```python
from build123d import *

# Parameters (mm, degrees)
SKETCH2_R           = 76.2
BOSS_EXTRUDE2_DEPTH = 76.2


with BuildPart() as part:
    # Sketch2 → Boss-Extrude2 (new body)
    with BuildSketch(Plane.XY):
        Polygon((0, 0), (803.656, 0), (549.615688221, -508), (131.991038362, -508), align=None)
        with Locations(Location((350.334210966, -312.584818641, 0), (0, 0, 180))):
            Circle(SKETCH2_R, mode=Mode.SUBTRACT)
    extrude(amount=BOSS_EXTRUDE2_DEPTH)


solid = part.part
```
Here's how the part is built. I have some questions about the finished solid (model axes, mm). Give positions to 0.01 mm unless a question says otherwise; leave off trailing zeros. Order: outer loops, then holes, each group sorted by start corner. A loop starts at its lowest first (then second) coordinate and runs counter-clockwise, first axis right, second up. Notation, with made-up numbers: (30, 30) - (71, 30) arc R27 ccw to (71, 50) - close; hole circle Ø4 at (73.5, 84.5). An arc over 180 degrees is marked (long way). Answer as a JSON object with one key per item and string values. Group by question number.
Item 1: For P1, Ø10, axis at y = -87, z = 10, coming from the -X side; P2, Ø4, axis at y = -345.5, z = 59, coming from the -X side; P3, Ø12, axis at y = -379, z = 34, coming from the -X side, each with a flat end and sliding along its axis, tell me the tip position at first contact or that it passes through.
Item 2: If we mould it in two halves opening along Y, with no side actions, what happens to faces 1 (the cylindrical face through (410.804, -266.218, 37.567)), 2 (the flat face through (396, 0, 38)), 3 (the flat face through (66.92, -257.56, 37.57))? For each: pulls with the +Y half, pulls with the -Y half, needs draft (parallel to the pull), parting line crosses it, or undercut.
Item 3: If we section it at C-C on x = 685: Please give me the cut outline in (y, z).
Item 4: If we section it at A-A on y = -248: Please give me the cut outline in (x, z), and give its area (3 significant figures).
Item 5: Please list where these lines run through material, in increasing order: probe 1 along Y at (x, z) = (354, 38); probe 2 along X at (y, z) = (-322, 34); probe 3 along X at (y, z) = (-304, 29.5).
Item 6: If we section it at B-B on z = 51: Please give me the cut outline in (x, y), and give its area (3 significant figures).
Item 7: If we section it at D-D on y = -54.5: Please give me the cut outline in (x, z), and give its area (3 significant figures).
Result set:
{
 "1": {"P1": "x = 21.31", "P2": "x = 89.25", "P3": "x = 96.91"},
 "2": {"face 1": "undercut", "face 2": "pulls with the +Y half", "face 3": "pulls with the -Y half"},
 "3": {"outline": "(-237.27, 0) - (0, 0) - (0, 76.2) - (-237.27, 76.2) - close"},
 "4": {"outline": "(64.44, 0) - (309.9, 0) - (309.9, 76.2) - (64.44, 76.2) - close; (390.77, 0) - (679.64, 0) - (679.64, 76.2) - (390.77, 76.2) - close", "area": "40,700 mm²"},
 "5": {"probe 1": "-508 to -388.7, -236.47 to 0", "probe 2": "83.66 to 274.72, 425.95 to 642.63", "probe 3": "78.99 to 274.62, 426.05 to 651.63"},
 "6": {"outline": "(0, 0) - (131.99, -508) - (549.62, -508) - (803.66, 0) - close; hole circle Ø152.4 at (350.33, -312.58)", "area": "292,000 mm²"},
 "7": {"outline": "(14.16, 0) - (776.4, 0) - (776.4, 76.2) - (14.16, 76.2) - close", "area": "58,100 mm²"}
}
